Model file for the job. Use its own axes, mm. Give positions to 0.01 mm unless a question says otherwise; leave off trailing zeros. Write each loop counter-clockwise with the first axis right and the second up, starting at its lowest first coordinate (ties: lowest second). Pieces come first, ordered by that corner, then holes.
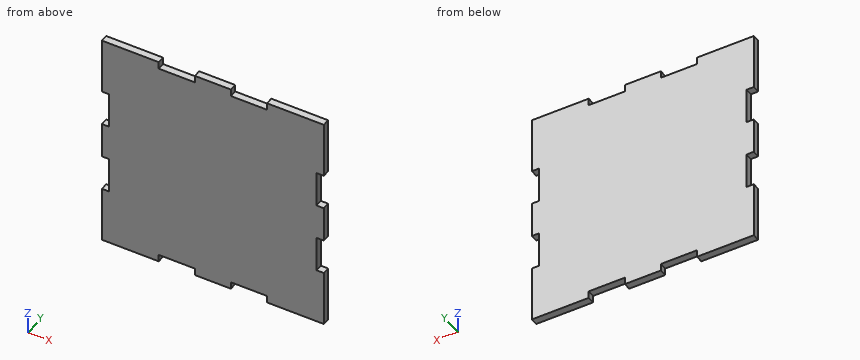
```python
from build123d import *

# Parameters (mm, degrees)
EXTRUDE_1_DEPTH = 4


with BuildPart() as part:
    # Эскиз1 → Бобышка-Вытянуть1 (new body)
    with BuildSketch(Plane(origin=(0, 0, 0), x_dir=(1, 0, 0), z_dir=(0, 1, 0))):
        Polygon((31.5, 0), (31.5, 4), (51.5, 4), (51.5, 0), (71.5, 0), (71.5, 4), (91.5, 4), (91.5, 0), (123, 0), (123, 31.5), (119, 31.5), (119, 51.5), (123, 51.5), (123, 71.5), (119, 71.5), (119, 91.5), (123, 91.5), (123, 123), (91.5, 123), (91.5, 119), (71.5, 119), (71.5, 123), (51.5, 123), (51.5, 119), (31.5, 119), (31.5, 123), (0, 123), (0, 91.5), (4, 91.5), (4, 71.5), (0, 71.5), (0, 51.5), (4, 51.5), (4, 31.5), (0, 31.5), (0, 0), align=None)
    extrude(amount=EXTRUDE_1_DEPTH)


solid = part.part
```
1. Slice it at B-B, the plane z = -44.5. Write the cut outline in (x, y), and give its area (3 significant figures).
Calculated:
outline: (4, 0) - (119, 0) - (119, 4) - (4, 4) - close
area: 460 mm2
2. Pin check, flat tips, straight feed: P1, Ø2, axis at x = 45, y = 2, coming from the +Z side; P2, Ø2, axis at x = 46.5, y = 2.5, coming from the -Z side. Stop position of each tip, or through.
Calculated:
P1: stops at z = -4
P2: stops at z = -119
3. Probe probe 1 along Z at (x, y) = (41.5, 2.65); probe 2 along X at (y, z) = (1.65, -42.5). List the from-to ranges inside material, lowest first.
Calculated:
probe 1: z = -119 to -4
probe 2: x = 4 to 119
4. Slice it at A-A, the plane x = 37. Write the cut outline in (y, z).
Calculated:
outline: (0, -119) - (4, -119) - (4, -4) - (0, -4) - close
